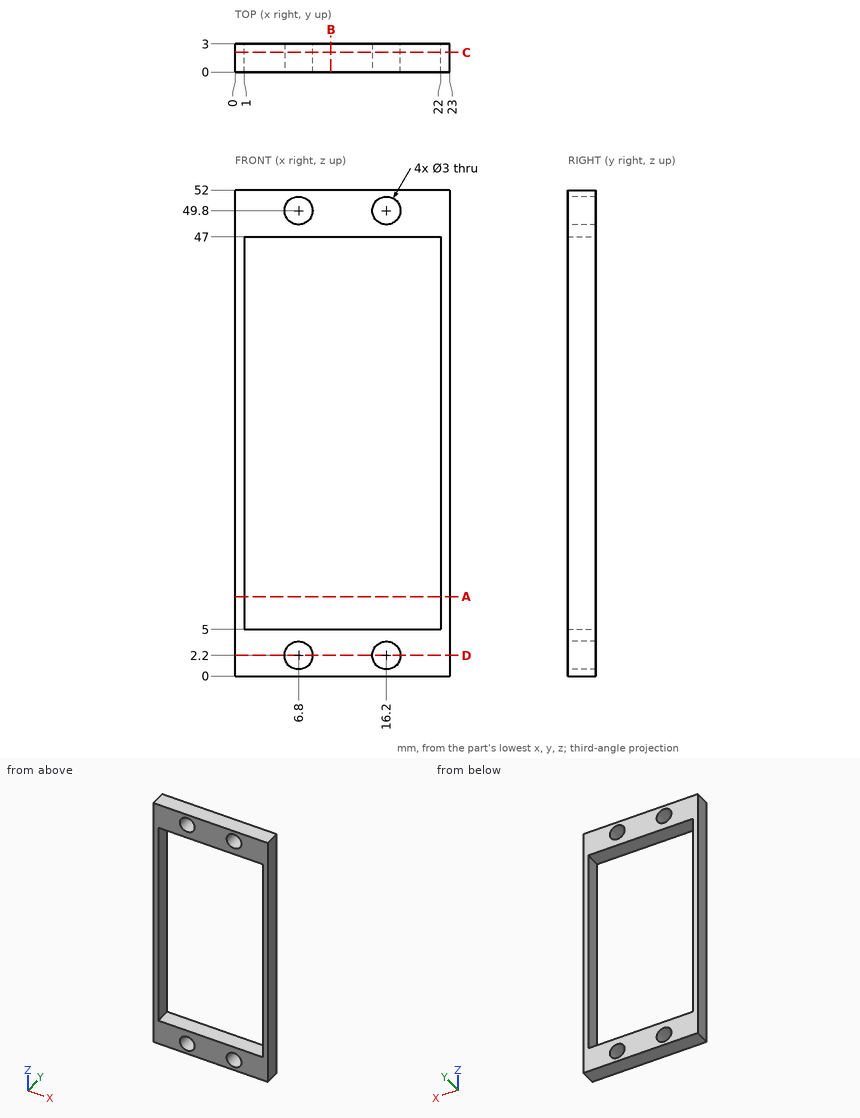
Verification items for this drawing (mm, ordinates from the low corner). Coordinates: 2 decimals unless noted, no trailing zeros. Order: outer loops, then holes, each group sorted by start corner. A loop starts at its lowest first (then second) coordinate and runs counter-clockwise, first axis right, second up. Notation, with made-up numbers: (-26.5, -16.75) - (-17.5, -16.75) arc R15 cw to (-17.5, -0.75) - close; hole circle Ø8 at (-13.5, 0.25). An arc over 180 degrees is marked (long way). Answer as a JSON object with one key per item and string values. Group by question number.
Item 1: Sectioned sample at C-C, the plane y = 2.1. Record the cut outline in (x, z), and give its area (3 significant figures).
Item 2: Sectioned sample at D-D, the plane z = 2.2. Record the cut outline in (x, y), and give its area (3 significant figures).
Item 3: Sectioned sample at B-B, the plane x = 10.25. Record the cut outline in (y, z).
Item 4: Depth check by flat-ended pin: pin 1 Ø1.5 at (x, y) = (10, 1.5) entering from -Z. Enter the tip coordinate at first touch or a pass-through.
Item 5: Sectioned sample at A-A, the plane z = 8.5. Record the cut outline in (x, y).
Item 6: Scan lines: probe 1 along Z at (x, y) = (16.2, 0.75); probe 2 along X at (y, z) = (1.8, 49.8); probe 3 along Z at (x, y) = (3.5, 0.9). Record each from-to range of solid material in increasing order.
Resolved:
{
 "1": {"outline": "(0, 0) - (23, 0) - (23, 52) - (0, 52) - close; hole (1, 5) - (22, 5) - (22, 47) - (1, 47) - close; hole circle Ø3 at (6.8, 2.2); hole circle Ø3 at (6.8, 49.8); hole circle Ø3 at (16.2, 2.2); hole circle Ø3 at (16.2, 49.8)", "area": "286 mm^2"},
 "2": {"outline": "(0, 0) - (5.3, 0) - (5.3, 3) - (0, 3) - close; (8.3, 0) - (14.7, 0) - (14.7, 3) - (8.3, 3) - close; (17.7, 0) - (23, 0) - (23, 3) - (17.7, 3) - close", "area": "51.0 mm^2"},
 "3": {"outline": "(0, 0) - (3, 0) - (3, 5) - (0, 5) - close; (0, 47) - (3, 47) - (3, 52) - (0, 52) - close"},
 "4": {"pin 1": "z = 0"},
 "5": {"outline": "(0, 0) - (1, 0) - (1, 3) - (0, 3) - close; (22, 0) - (23, 0) - (23, 3) - (22, 3) - close"},
 "6": {"probe 1": "0 to 0.7, 3.7 to 5, 47 to 48.3, 51.3 to 52", "probe 2": "0 to 5.3, 8.3 to 14.7, 17.7 to 23", "probe 3": "0 to 5, 47 to 52"}
}
